from build123d import *

# Parameters (mm, degrees)
F0_W     = 100
F0_H     = 100
F1_DEPTH = 100
F2_R     = 10
F2_R_2   = 9.5
F3_DEPTH = 30
F4_DEPTH = 100
F5_W     = 98
F5_H     = 98
F5_R     = 9.5
F6_DEPTH = 5


with BuildPart() as f1:
    # F0 (on Top) → F1 (new body)
    with BuildSketch(Plane.XY):
        Rectangle(F0_W, F0_H)
    extrude(amount=-F1_DEPTH)

    # F2 (on Top) → F3 (join)
    with BuildSketch(Plane.XY):
        Circle(F2_R)
        Circle(F2_R_2, mode=Mode.SUBTRACT)
    extrude(amount=F3_DEPTH)

    # F4 (cut, through all): a face of the model
    f4_faces = [f1.faces().sort_by_distance(p)[0] for p in [
        (0, 0, 0),
    ]]
    extrude(f4_faces, amount=-F4_DEPTH, mode=Mode.SUBTRACT)

    # F5 (on face) → F6 (cut)
    with BuildSketch(Plane(origin=(0, 0, -100), x_dir=(1, 0, 0), z_dir=(0, 0, -1))):
        Rectangle(F5_W, F5_H)
        Circle(F5_R, mode=Mode.SUBTRACT)
    extrude(amount=-F6_DEPTH, mode=Mode.SUBTRACT)


solid = f1.part
Input: part model. Units: mm. Frame: model coordinates. A direction names the side the tool comes from. Give positions to 0.01 mm unless a question says otherwise; leave off trailing zeros. Write each loop counter-clockwise with the first axis right and the second up, starting at its lowest first coordinate (ties: lowest second). Pieces come first, ordered by that corner, then holes. Notation, with made-up numbers: (-19.5, 42) -> (24.5, 42) arc R25 cw to (24.5, 63) -> close; hole circle Ø2 at (57, -39). An arc over 180 degrees is marked (long way). Use one line per item in the form item = value. Start each with the question number.
1) Section query C-C on z = -12. Return the cut outline in (x, y).
2) Section query A-A on x = 0. Return the cut outline in (y, z).
3) Pin query (flat end, axial travel): pin 1 (1 mm diameter, centred on x = 2, y = 12, fed in from -Z); pin 2 (1 mm diameter, centred on x = -31.5, y = 4.5, fed in from +Z); pin 3 (11.5 mm diameter, centred on x = 0, y = 0, fed in from +Z) (3 decimals). Return the tip coordinate at first contact, or that it passes through.
4) Draft query along X for faces 3 (the flat face through (10, -1, -95)), 4 (the cylindrical face through (-2.17, -9.76, 14.79)), 5 (the flat face through (-1, 12, 0)). Return one class per face: pulls with the +X half, pulls with the -X half, needs draft (parallel to the pull), parting line crosses it, or undercut.
5) Ray query, probe 1 along Y at (x, z) = (0, -47); probe 2 along Y at (x, z) = (0, 17.75); probe 3 along Z at (x, y) = (6, 35). Return the intervals inside material, ascending. Write a range as from..to.
6) Section query D-D on x = 15. Return the cut outline in (y, z), then the cut area to 3 significant figures.
7) Set-up query: faces 1 (the flat face through (-1, 49, -98)), 2 (the flat face through (-50, -1, -49)). Return all of +Z, -Z, +X, -X, +Y, -Y with unobstructed straight access to the full face (end or side cutting, diameter ignored); none if empty.
Outcome:
q1.outline = (-50, -50) -> (50, -50) -> (50, 50) -> (-50, 50) -> close; hole circle Ø19 at (0, 0)
q2.outline = (-50, -100) -> (-49, -100) -> (-49, -95) -> (-9.5, -95) -> (-9.5, 30) -> (-10, 30) -> (-10, 0) -> (-50, 0) -> close; (9.5, -95) -> (49, -95) -> (49, -100) -> (50, -100) -> (50, 0) -> (10, 0) -> (10, 30) -> (9.5, 30) -> close
q3.pin_1 = -95
q3.pin_2 = 0
q3.pin_3 = through
q4.face_3 = undercut
q4.face_4 = parting line crosses it
q4.face_5 = needs draft
q5.probe_1 = -50..-9.5, 9.5..50
q5.probe_2 = -10..-9.5, 9.5..10
q5.probe_3 = -95..0
q6.outline = (-50, -100) -> (-49, -100) -> (-49, -95) -> (49, -95) -> (49, -100) -> (50, -100) -> (50, 0) -> (-50, 0) -> close
q6.area = 9,510 mm^2
q7.face_1 = -Z
q7.face_2 = +Z, -Z, -X, +Y, -Y
